Read the model definition and answer for the solid it produces. Units are mm, in the model's axes. Face numbers are marked on the shaded views. A direction names the side the tool comes from. Give positions to 0.01 mm unless a question says otherwise; leave off trailing zeros. Order: outer loops, then holes, each group sorted by start corner. A loop starts at its lowest first (then second) coordinate and runs counter-clockwise, first axis right, second up. Notation, with made-up numbers: M 22,-16 L 72,-16 A10 cw 72,-11 Z; hole C 3,-40 d8. An arc over 180 degrees is marked long. One line per item, written item: value. Start each with the question number.
from build123d import *

# Parameters (mm, degrees)
BOSS_EXTRUDE1_DEPTH       = 25.4
F_6_CLEARANCE_HOLE1_D     = 3.7973
F_6_CLEARANCE_HOLE1_DEPTH = 12.7
F_6_CLEARANCE_HOLE1_TIP   = 1.140824014


with BuildPart() as part:
    # Sketch1 → Boss-Extrude1 (new body)
    with BuildSketch(Plane(origin=(0, 0, 0), x_dir=(1, 0, 0), z_dir=(0, 1, 0))):
        Polygon((-9.525, 10.998522628), (0, 10.998522628), (-9.525, -5.499261314), align=None)
        Polygon((9.525, -5.499261314), (0, 10.998522628), (-9.525, -5.499261314), align=None)
    extrude(amount=BOSS_EXTRUDE1_DEPTH)

    # #6 Clearance Hole1
    with Locations(Plane(origin=(0, 19.05, 5.499261314), x_dir=(1, 0, 0), z_dir=(0, 0, 1))):
        with Locations((0, 0), (0, -12.7)):
            Hole(F_6_CLEARANCE_HOLE1_D / 2, depth=F_6_CLEARANCE_HOLE1_DEPTH)
            with Locations((0, 0, -(F_6_CLEARANCE_HOLE1_DEPTH + F_6_CLEARANCE_HOLE1_TIP / 2))):  # 118° drill point
                Cone(0, F_6_CLEARANCE_HOLE1_D / 2, F_6_CLEARANCE_HOLE1_TIP, mode=Mode.SUBTRACT)


solid = part.part
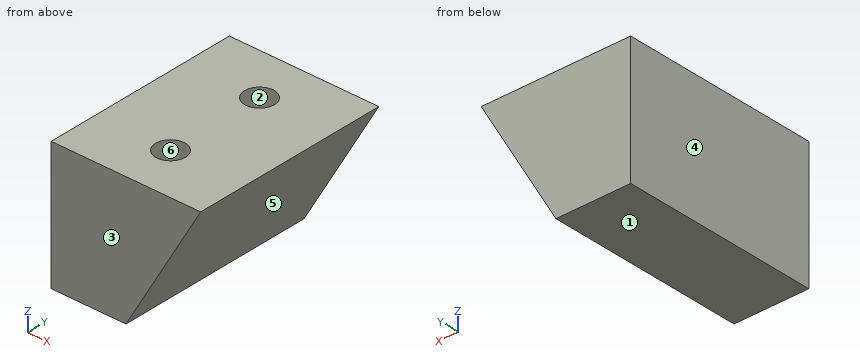
Q1. A tool of negligible diameter and unlimited length cuts with its end or side. For the marked faces 1 and 2, from which of +Z, -Z, +X, -X, +Y, -Y can it reach the whole face along a straight path? Write none if from no direction.
Q2. Find section C-C, the plane z = -4.5. Give the vertices of the cut face in (x, y) (3 decimals), then the cut area to 3 significant figures.
Q3. Determine the mould class of the marked faces 3, 4, 5 and 6 for opening direction X: released by +X, released by -X, zero draft, split by the parting line, or undercut.
Q4. Consider probe 1 along Y at (x, z) = (0, -2.75); probe 2 along Y at (x, z) = (-1.25, 0.75); probe 3 along X at (y, z) = (8, -2.5) (3 decimals). Determine where each line is inside the solid, lowest interval first.
Q5. Find section A-A, the plane z = 0. Give the vertices of the cut face in (x, y) (3 decimals).
Q6. Find section D-D, the plane x = 5.25. Give the vertices of the cut face in (y, z), then the cut area to 3 significant figures.
Q7. Find section B-B, the plane y = 23.25. Give the vertices of the cut face in (x, z) (3 decimals), then the cut area to 3 significant figures.
Evaluation:
1. face 1: -Z, +X, -X, +Y, -Y
1. face 2: +Z
2. outline: M -9.525,0 L 3.752,0 L 3.752,25.4 L -9.525,25.4 Z; hole C 0,6.35 d3.797; hole C 0,19.05 d3.797
2. area: 315 mm2
3. face 3: zero draft
3. face 4: released by -X
3. face 5: released by +X
3. face 6: undercut
4. probe 1: 0 to 4.45, 8.25 to 17.15, 20.95 to 25.4
4. probe 2: 0 to 4.92, 7.78 to 17.62, 20.48 to 25.4
4. probe 3: -9.525 to -0.939, 0.939 to 4.907
5. outline: M -9.525,0 L 6.35,0 L 6.35,25.4 L -9.525,25.4 Z; hole C 0,6.35 d3.797; hole C 0,19.05 d3.797
6. outline: M 0,-1.91 L 25.4,-1.91 L 25.4,5.5 L 0,5.5 Z
6. area: 188 mm2
7. outline: M -9.525,-10.999 L 0,-10.999 L 9.525,5.499 L -9.525,5.499 Z
7. area: 236 mm2
